Build history of the part. All positions in model axes, mm. Round coordinates to 2 decimals unless told otherwise and drop trailing zeros. Order: outer loops, then holes, each group sorted by start corner. A loop starts at its lowest first (then second) coordinate and runs counter-clockwise, first axis right, second up. Notation, with made-up numbers: M 85,-6 L 129,-6 A23 cw 129,10 Z; hole C 75.5,14 d2. An arc over 180 degrees is marked long. One line per item, written item: value. Start each with the question number.
Item 1: Band-saw the part on C-C, the plane x = 37. Write the cut outline in (y, z).
Item 2: Band-saw the part on B-B, the plane z = 4.25. Write the cut outline in (x, y), then the cut area to 3 significant figures.
Item 3: Pin check, flat tips, straight feed: pin 1 (3 mm diameter, centred on y = 52, z = 1.5, fed in from -X); pin 2 (1 mm diameter, centred on x = -6.5, z = 0.5, fed in from +Y); pin 3 (1 mm diameter, centred on x = 19, y = -42, fed in from -Z). Stop position of each tip, or through.
Item 4: Band-saw the part on D-D, the plane y = -52. Write the cut outline in (x, z), then the cut area to 3 significant figures.
Item 5: Probe L1, parallel to Z at x = 19, y = 71; L2, parallel to Y at x = 23, z = 2.45; L3, parallel to X at y = 9, z = 1.65. List the from-to ranges inside material, lowest first.
Item 6: Band-saw the part on A-A, the plane y = 27. Write the cut outline in (x, z), then the cut area to 3 significant figures.
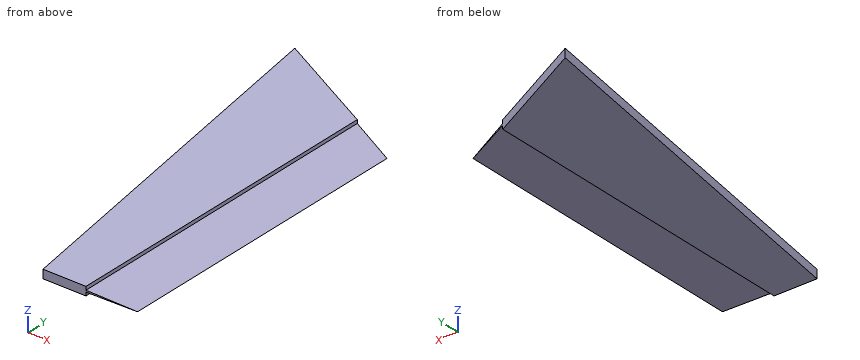
```python
from build123d import *

# Parameters (mm, degrees)
EXTRUDE_1_DEPTH     = 5
CUT_EXTRUDE_2_DEPTH = 200


with BuildPart() as part:
    # 草图1 → 凸台-拉伸1 (new body)
    with BuildSketch(Plane.XY):
        Polygon((-7.259084377, -114.381441925), (-45.249305145, 114.381441925), (47.740915623, 65.618558075), (47.740915623, -114.381441925), align=None)
    extrude(amount=EXTRUDE_1_DEPTH)

    # 草图2 → 切除-拉伸2 (cut)
    with BuildSketch(Plane.XZ.offset(114.381441925)):
        Polygon((17.740915623, 5), (47.740915623, 5.362068385), (52.130743892, 0.972240116), (47.740915623, -0.81389846), (17.740915623, 0), (17.740915623, 1.999597824), (47.740915623, 2.5), (17.740915623, 3.000402176), align=None)
        Polygon((47.740915623, 35.362068385), (52.130743892, 30.972240116), (47.740915623, 29.18610154), (17.740915623, 30), (17.740915623, 31.999597824), (47.740915623, 32.5), (17.740915623, 33.000402176), (17.740915623, 35), align=None)
    extrude(amount=-CUT_EXTRUDE_2_DEPTH, mode=Mode.SUBTRACT)


solid = part.part
```
Output:
1. outline: M -114.38,2.32 L 71.25,2.32 L 71.25,2.68 L -114.38,2.68 Z
2. outline: M -45.25,114.38 L -7.26,-114.38 L 17.74,-114.38 L 17.74,81.35 Z
2. area: 9,020 mm²
3. pin 1: stops at x = -35.14
3. pin 2: stops at y = 94.32
3. pin 3: stops at z = 2.01
4. outline: M -17.62,0 L 17.74,0 L 17.74,2 L 47.74,2.5 L 17.74,3 L 17.74,5 L -17.62,5 Z
4. area: 192 mm²
5. L1: z = 2.02 to 2.98
5. L2: y = -114.38 to 78.59
5. L3: x = -27.75 to 17.74
6. outline: M -30.74,0 L 17.74,0 L 17.74,2 L 47.74,2.5 L 17.74,3 L 17.74,5 L -30.74,5 Z
6. area: 257 mm²
